CAD build for the part. Positions are in the model's coordinates, mm. Face numbers are marked on the shaded views. A direction names the side the tool comes from. Coordinates: 2 decimals unless noted, no trailing zeros. Write each loop counter-clockwise with the first axis right and the second up, starting at its lowest first coordinate (ties: lowest second). Pieces come first, ordered by that corner, then holes. Notation, with made-up numbers: (14.5, 28.25) - (28.5, 28.25) arc R19 cw to (28.5, 64.25) - close; hole circle Ø3 at (22, 81). An arc over 180 degrees is marked (long way). Answer in a Markdown table with one row per item. Add a question column.
Q1. Drill centre lines: line 1 along X through (y, z) = (-3.5, 10.5); line 2 along Z through (x, y) = (4, 0.5); line 3 along X through (y, z) = (1.5, 3.75). Where is each one in solid material? Low to high. Write a range as from..to.
Q2. Band-saw the part on C-C (x = 0). List the corners of the cut face in (y, z).
Q3. Band-saw the part on A-A (y = 0). List the corners of the cut face in (x, z).
Q4. Band-saw the part on B-B (z = 10.75). List the corners of the cut face in (x, y), and give its area (3 significant figures).
Q5. Pin check, flat tips, straight feed: pin 1 (2 mm diameter, centred on x = 3, z = 6.5, fed in from -Y); pin 2 (1.5 mm diameter, centred on y = -0.5, z = 14, fed in from -X); pin 3 (2 mm diameter, centred on x = -2.5, z = 2.5, fed in from +Y). Stop position of each tip, or through.
Q6. Band-saw the part on D-D (z = 3). List the corners of the cut face in (x, y).
Q7. 3-axis set-ups, long thin cutter, end or side, ignore diameter. For the marked faces 1, 2, 3 and 4: which of +Z, -Z, +X, -X, +Y, -Y reach the whole face in a straight line?
```python
from build123d import *

# Parameters (mm, degrees)
SKETCH_1_R          = 3.3
EXTRUDE_1_DEPTH     = 8
SKETCH_2_R          = 4
EXTRUDE_2_DEPTH     = 4.2
SKETCH_3_R          = 4.5
EXTRUDE_3_DEPTH     = 1
SKETCH_4_OUTSIDE_W  = 18.132
SKETCH_4_OUTSIDE_H  = 18.132
SKETCH_4_OUTSIDE_R  = 4.155576512
CUT_EXTRUDE_1_DEPTH = 1
CUT_EXTRUDE_1_DRAFT = -60
EXTRUDE_4_DEPTH     = 3
SKETCH_6_OUTSIDE_W  = 25.512
SKETCH_6_OUTSIDE_H  = 25.512
SKETCH_6_OUTSIDE_R  = 3.481100129
CUT_EXTRUDE_2_DEPTH = 3
CUT_EXTRUDE_2_DRAFT = -60
CHAMFER_1_SIZE      = 1


with BuildPart() as part:
    # Sketch 1 → Extrude 1 (new body)
    with BuildSketch(Plane.XY):
        Circle(SKETCH_1_R)
    extrude(amount=EXTRUDE_1_DEPTH)

    # Sketch 2 → Extrude 2 (add)
    with BuildSketch(Plane.XY.offset(8)):
        Circle(SKETCH_2_R)
    extrude(amount=EXTRUDE_2_DEPTH)

    # Sketch 3 → Extrude 3 (add)
    with BuildSketch(Plane.XY.offset(12.2)):
        Circle(SKETCH_3_R)
    extrude(amount=EXTRUDE_3_DEPTH)


with BuildPart() as cut_extrude_1_tool:
    # Sketch 4 outside → Cut-Extrude 1 (with draft: the straight prism first)
    with BuildSketch(Plane.XY.offset(13.2)):
        Rectangle(SKETCH_4_OUTSIDE_W, SKETCH_4_OUTSIDE_H)
        Circle(SKETCH_4_OUTSIDE_R, mode=Mode.SUBTRACT)
    extrude(amount=-CUT_EXTRUDE_1_DEPTH)
    # Cut-Extrude 1: the draft: its side faces are tilted about the plane it starts from
    cut_extrude_1_sides = [cut_extrude_1_tool.faces().sort_by_distance(p)[0] for p in [
        (0, -9.066, 12.7),
        (9.066, 0, 12.7),
        (0, 9.066, 12.7),
        (-9.066, 0, 12.7),
        (-4.155576512, 0, 12.7),
    ]]
    draft(cut_extrude_1_sides, Plane.XY.offset(13.2), CUT_EXTRUDE_1_DRAFT)


with BuildPart() as part_1:
    add(part.part)

    # Cut-Extrude 1: cut by cut_extrude_1_tool
    add(cut_extrude_1_tool.part, mode=Mode.SUBTRACT)

    # Sketch 5 → Extrude 4 (add)
    with BuildSketch(Plane.XY.offset(13.2)):
        Polygon((-4.152198442, 0.167523856), (-2.221179136, -3.512147404), (1.931019306, -3.679671261), (4.152198442, -0.167523856), (2.221179136, 3.512147404), (-1.931019306, 3.679671261), align=None)
    extrude(amount=EXTRUDE_4_DEPTH)


with BuildPart() as cut_extrude_2_tool:
    # Sketch 6 outside → Cut-Extrude 2 (with draft: the straight prism first)
    with BuildSketch(Plane.XY.offset(16.2)):
        Rectangle(SKETCH_6_OUTSIDE_W, SKETCH_6_OUTSIDE_H)
        Circle(SKETCH_6_OUTSIDE_R, mode=Mode.SUBTRACT)
    extrude(amount=-CUT_EXTRUDE_2_DEPTH)
    # Cut-Extrude 2: the draft: its side faces are tilted about the plane it starts from
    cut_extrude_2_sides = [cut_extrude_2_tool.faces().sort_by_distance(p)[0] for p in [
        (0, -12.756, 14.7),
        (12.756, 0, 14.7),
        (0, 12.756, 14.7),
        (-12.756, 0, 14.7),
        (-3.481100129, 0, 14.7),
    ]]
    draft(cut_extrude_2_sides, Plane.XY.offset(16.2), CUT_EXTRUDE_2_DRAFT)


with BuildPart() as part_2:
    add(part_1.part)

    # Cut-Extrude 2: cut by cut_extrude_2_tool
    add(cut_extrude_2_tool.part, mode=Mode.SUBTRACT)

    # Chamfer 1
    chamfer_1_edges = [part_2.edges().sort_by_distance(p)[0] for p in [
        (-3.3, 0, 0),
    ]]
    chamfer(chamfer_1_edges, length=CHAMFER_1_SIZE)


solid = part_2.part
```
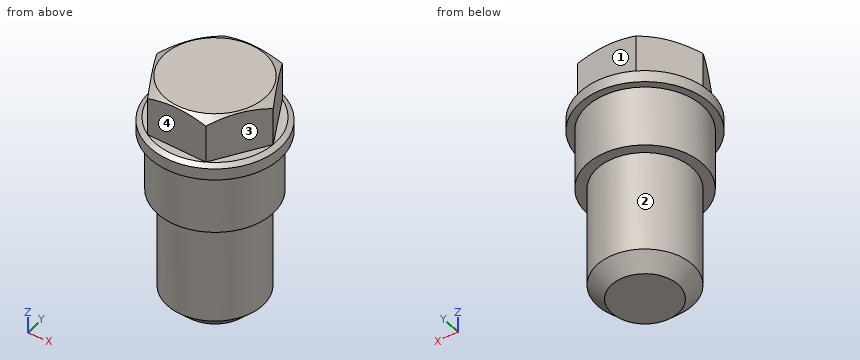
Checked values:
| question | item | result |
|---|---|---|
| 1 | line 1 | x = -1.94..1.94 |
| 1 | line 2 | z = 12.2..13.2 |
| 1 | line 3 | x = -2.94..2.94 |
| 2 | outline | (-4.5, 12.2) - (-4, 12.2) - (-4, 8) - (-3.3, 8) - (-3.3, 1) - (-2.3, 0) - (2.3, 0) - (3.3, 1) - (3.3, 8) - (4, 8) - (4, 12.2) - (4.5, 12.2) - (4.5, 13) - (4.16, 13.2) - (3.6, 13.2) - (3.6, 16.13) - (3.48, 16.2) - (-3.48, 16.2) - (-3.6, 16.13) - (-3.6, 13.2) - (-4.16, 13.2) - (-4.5, 13) - close |
| 3 | outline | (-4.5, 12.2) - (-4, 12.2) - (-4, 8) - (-3.3, 8) - (-3.3, 1) - (-2.3, 0) - (2.3, 0) - (3.3, 1) - (3.3, 8) - (4, 8) - (4, 12.2) - (4.5, 12.2) - (4.5, 13) - (4.16, 13.2) - (4.06, 13.2) - (4.06, 15.86) - (3.48, 16.2) - (-3.48, 16.2) - (-4.06, 15.86) - (-4.06, 13.2) - (-4.16, 13.2) - (-4.5, 13) - close |
| 4 | outline | circle Ø8 at (0, 0) |
| 4 | area | 50.3 mm² |
| 5 | pin 1 | stops at y = -2.62 |
| 5 | pin 2 | stops at x = -4.15 |
| 5 | pin 3 | stops at y = 2.94 |
| 6 | outline | circle Ø6.6 at (0, 0) |
| 7 | face 1 | +Z, +X, +Y |
| 7 | face 2 | -Z |
| 7 | face 3 | +Z, +X, -Y |
| 7 | face 4 | +Z, -X, -Y |
